Design review of the part built by this model. Coordinates are the model's own, in mm. Face numbers are marked on the shaded views. A direction names the side the tool comes from. Coordinates: 2 decimals unless noted, no trailing zeros. Write each loop counter-clockwise with the first axis right and the second up, starting at its lowest first coordinate (ties: lowest second). Pieces come first, ordered by that corner, then holes.
Q1. Add section D-D, the plane y = -4.55. Give the boundary of the cut face in (x, z), plus the area to 3 significant figures.
Q2. Machinability: for the marked faces 1, 2, 3, 4 and 5, which of the approach directions +Z, -Z, +X, -X, +Y, -Y give a long, thin tool a straight path to every point of the face, cutting with its end or side? Answer none if there is none.
Q3. The part is to be moulded in two halves that separate along X. For the marked faces 6, 7 and 8, say which applies: +X half, -X half, draft (parallel to the pull), parting line (faces both ways), or undercut.
Q4. Clearance check with flat-ended pins moving along their axes: pin 1 Ø1.2 at (x, z) = (6.5, 0) entering from +Y; pin 2 Ø2 at (x, z) = (-2, -1) entering from -Y; pin 3 Ø1 at (y, z) = (16, -1.5) entering from +X. State where each tip first meets the part, or that it passes through.
Q5. To check wall thickness, follow probe 1 along Y at (x, z) = (7, 1.8); probe 2 along X at (y, z) = (2.5, -1.65); probe 3 along X at (y, z) = (17, -1.55). State the ranges of each line that lie inside material, in increasing order.
Q6. Add section C-C, the plane x = 6.5. Give the boundary of the cut face in (y, z), plus the area to 3 significant figures.
Q7. Add section A-A, the plane x = -12.5. Give the boundary of the cut face in (y, z), plus the area to 3 significant figures.
Q8. Add section B-B, the plane y = 17.5. Give the boundary of the cut face in (x, z), plus the area to 3 significant figures.
from build123d import *

# Parameters (mm, degrees)
BOSS_EXTRU_1_DEPTH = 2
CONG_1_R           = 2


with BuildPart() as part:
    # Esquisse1 → Boss.-Extru.1 (new body, symmetric)
    with BuildSketch(Plane.XY):
        Polygon((-17.5, -25), (-17.5, 25), (-7.5, 25), (-7.5, 11.25), (17.5, 11.25), (17.5, -11.25), (-7.5, -11.25), (-7.5, -25), align=None)
        with BuildLine():
            Line((3.2, 6.25), (13.8, 6.25))
            ThreePointArc((13.8, 6.25), (15.5, 4.55), (13.8, 2.85))
            Line((13.8, 2.85), (3.2, 2.85))
            ThreePointArc((3.2, 2.85), (1.5, 4.55), (3.2, 6.25))
        make_face(mode=Mode.SUBTRACT)
        with BuildLine():
            Line((3.2, -6.25), (13.8, -6.25))
            ThreePointArc((13.8, -6.25), (15.5, -4.55), (13.8, -2.85))
            Line((13.8, -2.85), (3.2, -2.85))
            ThreePointArc((3.2, -2.85), (1.5, -4.55), (3.2, -6.25))
        make_face(mode=Mode.SUBTRACT)
        with BuildLine():
            Line((-10.8, 20), (-10.8, -20))
            ThreePointArc((-10.8, -20), (-12.5, -21.7), (-14.2, -20))
            Line((-14.2, -20), (-14.2, 20))
            ThreePointArc((-14.2, 20), (-12.5, 21.7), (-10.8, 20))
        make_face(mode=Mode.SUBTRACT)
    extrude(amount=BOSS_EXTRU_1_DEPTH, both=True)

    # Congé1
    cong_1_edges = [part.edges().sort_by_distance(p)[0] for p in [
        (-17.5, -25, 0),
        (-17.5, 25, 0),
        (-7.5, 25, 0),
        (-7.5, 11.25, 0),
        (17.5, 11.25, 0),
        (17.5, -11.25, 0),
        (-7.5, -11.25, 0),
        (-7.5, -25, 0),
    ]]
    fillet(cong_1_edges, radius=CONG_1_R)


solid = part.part
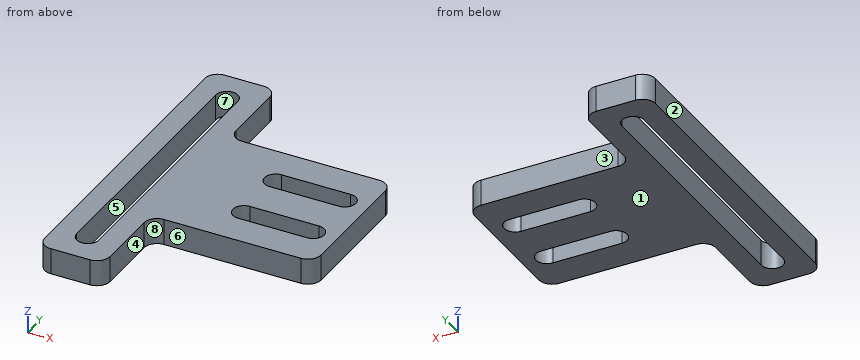
Here are the results:
1. outline: (-17.5, -2) - (-14.2, -2) - (-14.2, 2) - (-17.5, 2) - close; (-10.8, -2) - (1.5, -2) - (1.5, 2) - (-10.8, 2) - close; (15.5, -2) - (17.5, -2) - (17.5, 2) - (15.5, 2) - close
1. area: 70.4 mm2
2. face 1: -Z, +X, -X, +Y, -Y
2. face 2: +Z, -Z, -X, +Y, -Y
2. face 3: +Z, -Z, +X, +Y
2. face 4: +Z, -Z, +X, -Y
2. face 5: +Z, -Z
3. face 6: draft
3. face 7: undercut
3. face 8: +X half
4. pin 1: stops at y = 11.25
4. pin 2: stops at y = -11.25
4. pin 3: stops at x = -7.5
5. probe 1: y = -11.25 to -6.25, -2.85 to 2.85, 6.25 to 11.25
5. probe 2: x = -17.5 to -14.2, -10.8 to 17.5
5. probe 3: x = -17.5 to -14.2, -10.8 to -7.5
6. outline: (-11.25, -2) - (-6.25, -2) - (-6.25, 2) - (-11.25, 2) - close; (-2.85, -2) - (2.85, -2) - (2.85, 2) - (-2.85, 2) - close; (6.25, -2) - (11.25, -2) - (11.25, 2) - (6.25, 2) - close
6. area: 62.8 mm2
7. outline: (-25, -2) - (-21.7, -2) - (-21.7, 2) - (-25, 2) - close; (21.7, -2) - (25, -2) - (25, 2) - (21.7, 2) - close
7. area: 26.4 mm2
8. outline: (-17.5, -2) - (-14.2, -2) - (-14.2, 2) - (-17.5, 2) - close; (-10.8, -2) - (-7.5, -2) - (-7.5, 2) - (-10.8, 2) - close
8. area: 26.4 mm2
